from build123d import *

# Parameters (mm, degrees)
SKETCH1_R           = 11.1
BOSS_EXTRUDE1_DEPTH = 8
SKETCH2_R           = 42.5
SKETCH2_R_2         = 15
BOSS_EXTRUDE2_DEPTH = 2
FILLET1_R           = 1.5


with BuildPart() as part:
    # Sketch1 → Boss-Extrude1 (new body, symmetric)
    with BuildSketch(Plane(origin=(0, 0, 0), x_dir=(1, 0, 0), z_dir=(0, 1, 0))):
        with BuildLine():
            ThreePointArc((39.96011477, -3.097680993), (36.98, 0), (39.96011477, 3.097680993))
            ThreePointArc((39.96011477, 3.097680993), (39.887003845, 3.928526984), (39.796619952, 4.757671737))
            ThreePointArc((39.796619952, 4.757671737), (36.269439669, 7.214440108), (38.587964788, 10.833991579))
            ThreePointArc((38.587964788, 10.833991579), (38.354168656, 11.634609864), (38.103763348, 12.430189811))
            ThreePointArc((38.103763348, 12.430189811), (34.165065112, 14.151633329), (35.732900959, 18.153957945))
            ThreePointArc((35.732900959, 18.153957945), (35.347404275, 18.893581212), (34.946600487, 19.625022661))
            ThreePointArc((34.946600487, 19.625022661), (30.747746263, 20.544987217), (31.504641785, 24.776277888))
            ThreePointArc((31.504641785, 24.776277888), (30.982258971, 25.426482829), (30.446459367, 26.065676895))
            ThreePointArc((30.446459367, 26.065676895), (26.148808768, 26.148808768), (26.065676895, 30.446459367))
            ThreePointArc((26.065676895, 30.446459367), (25.426482829, 30.982258971), (24.776277888, 31.504641785))
            ThreePointArc((24.776277888, 31.504641785), (20.544987217, 30.747746263), (19.625022661, 34.946600487))
            ThreePointArc((19.625022661, 34.946600487), (18.893581212, 35.347404275), (18.153957945, 35.732900959))
            ThreePointArc((18.153957945, 35.732900959), (14.151633329, 34.165065112), (12.430189811, 38.103763348))
            ThreePointArc((12.430189811, 38.103763348), (11.634609864, 38.354168656), (10.833991579, 38.587964788))
            ThreePointArc((10.833991579, 38.587964788), (7.214440108, 36.269439669), (4.757671737, 39.796619952))
            ThreePointArc((4.757671737, 39.796619952), (3.928526984, 39.887003845), (3.097680993, 39.96011477))
            ThreePointArc((3.097680993, 39.96011477), (0, 36.98), (-3.097680993, 39.96011477))
            ThreePointArc((-3.097680993, 39.96011477), (-3.928526984, 39.887003845), (-4.757671737, 39.796619952))
            ThreePointArc((-4.757671737, 39.796619952), (-7.214440108, 36.269439669), (-10.833991579, 38.587964788))
            ThreePointArc((-10.833991579, 38.587964788), (-11.634609864, 38.354168656), (-12.430189811, 38.103763348))
            ThreePointArc((-12.430189811, 38.103763348), (-14.151633329, 34.165065112), (-18.153957945, 35.732900959))
            ThreePointArc((-18.153957945, 35.732900959), (-18.893581212, 35.347404275), (-19.625022661, 34.946600487))
            ThreePointArc((-19.625022661, 34.946600487), (-20.544987217, 30.747746263), (-24.776277888, 31.504641785))
            ThreePointArc((-24.776277888, 31.504641785), (-25.426482829, 30.982258971), (-26.065676895, 30.446459367))
            ThreePointArc((-26.065676895, 30.446459367), (-26.148808768, 26.148808768), (-30.446459367, 26.065676895))
            ThreePointArc((-30.446459367, 26.065676895), (-30.982258971, 25.426482829), (-31.504641785, 24.776277888))
            ThreePointArc((-31.504641785, 24.776277888), (-30.747746263, 20.544987217), (-34.946600487, 19.625022661))
            ThreePointArc((-34.946600487, 19.625022661), (-35.347404275, 18.893581212), (-35.732900959, 18.153957945))
            ThreePointArc((-35.732900959, 18.153957945), (-34.165065112, 14.151633329), (-38.103763348, 12.430189811))
            ThreePointArc((-38.103763348, 12.430189811), (-38.354168656, 11.634609864), (-38.587964788, 10.833991579))
            ThreePointArc((-38.587964788, 10.833991579), (-36.269439669, 7.214440108), (-39.796619952, 4.757671737))
            ThreePointArc((-39.796619952, 4.757671737), (-39.887003845, 3.928526984), (-39.96011477, 3.097680993))
            ThreePointArc((-39.96011477, 3.097680993), (-36.98, 0), (-39.96011477, -3.097680993))
            ThreePointArc((-39.96011477, -3.097680993), (-39.887003845, -3.928526984), (-39.796619952, -4.757671737))
            ThreePointArc((-39.796619952, -4.757671737), (-36.269439669, -7.214440108), (-38.587964788, -10.833991579))
            ThreePointArc((-38.587964788, -10.833991579), (-38.354168656, -11.634609864), (-38.103763348, -12.430189811))
            ThreePointArc((-38.103763348, -12.430189811), (-34.165065112, -14.151633329), (-35.732900959, -18.153957945))
            ThreePointArc((-35.732900959, -18.153957945), (-35.347404275, -18.893581212), (-34.946600487, -19.625022661))
            ThreePointArc((-34.946600487, -19.625022661), (-30.747746263, -20.544987217), (-31.504641785, -24.776277888))
            ThreePointArc((-31.504641785, -24.776277888), (-30.982258971, -25.426482829), (-30.446459367, -26.065676895))
            ThreePointArc((-30.446459367, -26.065676895), (-26.148808768, -26.148808768), (-26.065676895, -30.446459367))
            ThreePointArc((-26.065676895, -30.446459367), (-25.426482829, -30.982258971), (-24.776277888, -31.504641785))
            ThreePointArc((-24.776277888, -31.504641785), (-20.544987217, -30.747746263), (-19.625022661, -34.946600487))
            ThreePointArc((-19.625022661, -34.946600487), (-18.893581212, -35.347404275), (-18.153957945, -35.732900959))
            ThreePointArc((-18.153957945, -35.732900959), (-14.151633329, -34.165065112), (-12.430189811, -38.103763348))
            ThreePointArc((-12.430189811, -38.103763348), (-11.634609864, -38.354168656), (-10.833991579, -38.587964788))
            ThreePointArc((-10.833991579, -38.587964788), (-7.214440108, -36.269439669), (-4.757671737, -39.796619952))
            ThreePointArc((-4.757671737, -39.796619952), (-3.928526984, -39.887003845), (-3.097680993, -39.96011477))
            ThreePointArc((-3.097680993, -39.96011477), (0, -36.98), (3.097680993, -39.96011477))
            ThreePointArc((3.097680993, -39.96011477), (3.928526984, -39.887003845), (4.757671737, -39.796619952))
            ThreePointArc((4.757671737, -39.796619952), (7.214440108, -36.269439669), (10.833991579, -38.587964788))
            ThreePointArc((10.833991579, -38.587964788), (11.634609864, -38.354168656), (12.430189811, -38.103763348))
            ThreePointArc((12.430189811, -38.103763348), (14.151633329, -34.165065112), (18.153957945, -35.732900959))
            ThreePointArc((18.153957945, -35.732900959), (18.893581212, -35.347404275), (19.625022661, -34.946600487))
            ThreePointArc((19.625022661, -34.946600487), (20.544987217, -30.747746263), (24.776277888, -31.504641785))
            ThreePointArc((24.776277888, -31.504641785), (25.426482829, -30.982258971), (26.065676895, -30.446459367))
            ThreePointArc((26.065676895, -30.446459367), (26.148808768, -26.148808768), (30.446459367, -26.065676895))
            ThreePointArc((30.446459367, -26.065676895), (30.982258971, -25.426482829), (31.504641785, -24.776277888))
            ThreePointArc((31.504641785, -24.776277888), (30.747746263, -20.544987217), (34.946600487, -19.625022661))
            ThreePointArc((34.946600487, -19.625022661), (35.347404275, -18.893581212), (35.732900959, -18.153957945))
            ThreePointArc((35.732900959, -18.153957945), (34.165065112, -14.151633329), (38.103763348, -12.430189811))
            ThreePointArc((38.103763348, -12.430189811), (38.354168656, -11.634609864), (38.587964788, -10.833991579))
            ThreePointArc((38.587964788, -10.833991579), (36.269439669, -7.214440108), (39.796619952, -4.757671737))
            ThreePointArc((39.796619952, -4.757671737), (39.887003845, -3.928526984), (39.96011477, -3.097680993))
        make_face()
        Circle(SKETCH1_R, mode=Mode.SUBTRACT)
    extrude(amount=BOSS_EXTRUDE1_DEPTH, both=True)

    # Sketch2 → Boss-Extrude2 (add)
    with BuildSketch(Plane(origin=(0, 8, 0), x_dir=(1, 0, 0), z_dir=(0, 1, 0))):
        Circle(SKETCH2_R)
        Circle(SKETCH2_R_2, mode=Mode.SUBTRACT)
    boss_extrude2 = extrude(amount=BOSS_EXTRUDE2_DEPTH)

    # Mirror1: Boss-Extrude2 across plane
    add(boss_extrude2.mirror(Plane.ZX))

    # Fillet1
    fillet1_edges = [part.edges().sort_by_distance(p)[0] for p in [
        (-42.5, 8, 0),
        (-42.5, -8, 0),
    ]]
    fillet(fillet1_edges, radius=FILLET1_R)


solid = part.part
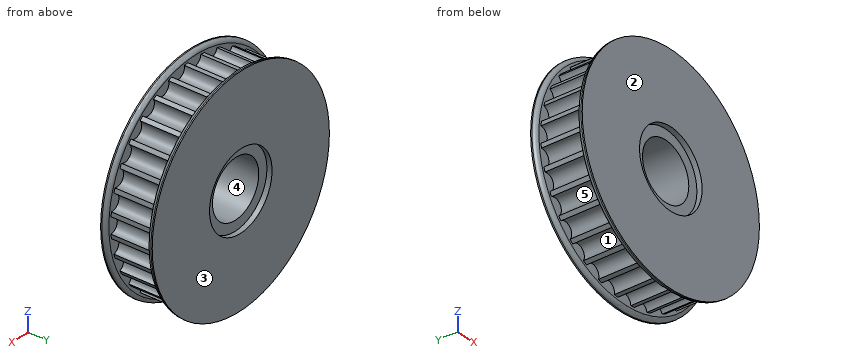
Geometry: final body of the model. Coordinates: model frame, mm. Face numbers are marked on the shaded views. A direction names the side the tool comes from. Give positions to 0.01 mm unless a question says otherwise; leave off trailing zeros. Loops run counter-clockwise (first coordinate to the right, second up) from the corner with the lowest first, then second, coordinate; pieces in that order, holes last. Notation, with made-up numbers: (21.25, 54.5) - (37.25, 54.5) arc R22 ccw to (37.25, 86.5) - close; hole circle Ø11 at (29, 79). An arc over 180 degrees is marked (long way). Answer as CSV lines item,"result". Start each with the question number.
1. Draft query along Y for the marked faces 1, 2 and 3. Return one class per face: released by +Y, released by -Y, zero draft, split by the parting line, or undercut.
2. Section A-A, the plane x = 0. Return loops of the section in (y, z).
3. Reachability of the marked faces 4 and 5 from +Z, -Z, +X, -X, +Y, -Y: full face, straight path, thin tool, end or side. Return the list, or none.
4. Ray query, L1, parallel to Z at x = 0, y = 3.25; L2, parallel to X at y = -9.4, z = 0; L3, parallel to X at y = -6.5, z = 31. Return the intervals inside material, ascending.
5. Pin query (flat end, axial travel): P1, Ø3, axis at x = -32, y = -1, coming from the -Z side; P2, Ø9, axis at x = 7.5, z = -4, coming from the -Y side; P3, Ø4, axis at y = -0.5, z = -28, coming from the -X side; P4, Ø24, axis at x = 0.5, z = 3, coming from the +Y side. Return the tip coordinate at first contact, or that it passes through.
Answers:
1,face 1,"undercut"
1,face 2,"released by -Y"
1,face 3,"released by +Y"
2,outline,"(-10, -42.5) - (-9.5, -42.5) arc R1.5 ccw to (-8, -41) - (-8, -36.98) - (8, -36.98) - (8, -41) arc R1.5 ccw to (9.5, -42.5) - (10, -42.5) - (10, -15) - (8, -15) - (8, -11.1) - (-8, -11.1) - (-8, -15) - (-10, -15) - close; (-10, 15) - (-8, 15) - (-8, 11.1) - (8, 11.1) - (8, 15) - (10, 15) - (10, 42.5) - (9.5, 42.5) arc R1.5 ccw to (8, 41) - (8, 36.98) - (-8, 36.98) - (-8, 41) arc R1.5 ccw to (-9.5, 42.5) - (-10, 42.5) - close"
3,face 4,"+Y, -Y"
3,face 5,"none"
4,L1,"z = -36.98 to -11.1, 11.1 to 36.98"
4,L2,"x = -42.5 to -15, 15 to 42.5"
4,L3,"x = -25.4 to -24.32, -20.22 to 20.22, 24.32 to 25.4"
5,P1,"stops at z = -26"
5,P2,"stops at y = -8"
5,P3,"stops at x = -30.5"
5,P4,"stops at y = 10"
